CAD build for the part. Positions are in the model's coordinates, mm. A direction names the side the tool comes from. Coordinates: 2 decimals unless noted, no trailing zeros. Loops run counter-clockwise (first coordinate to the right, second up) from the corner with the lowest first, then second, coordinate; pieces in that order, holes last. Notation, with made-up numbers: M 12,82 L 39,82 A5 cw 39,91 Z; hole C 82.25,-30.5 d7. An arc over 180 degrees is marked long. Answer as a JSON object with one key per item and string values. Group by question number.
Solid Edge part; units mm, degrees
sketch "Sketch1" plane through (0, 0, 0) normal (0, -1, 0) x (1, 0, 0)
  line L0 (139.7, 114.3) -> (-139.7, 114.3)
  line L1 (-139.7, 114.3) -> (-139.7, -114.3)
  line L2 (-139.7, -114.3) -> (139.7, -114.3)
  line L3 (139.7, -114.3) -> (139.7, 114.3)
extrude "Protrusion1" add sketch "Sketch1" against normal blind 158.75
shell "Thinwall_1" thickness 38.1 removed faces 1 at (-90.3393, 0, 78.486)
Item 1: Slice it at B-B, the plane z = -41. Write the cut outline in (x, y).
Item 2: Pull direction Z, two halves, no side cores. Call faces 1 (the flat face through (2, 158.75, 2)), 2 (the flat face through (2, 78, 114.3)), 3 (the flat face through (101.6, 59, -1)): released by +Z, released by -Z, zero draft, split by the parting line, or undercut.
Item 3: Tool access for faces 4 (the flat face through (-1, 59, -76.2)), 5 (the flat face through (-2, 78, -114.3)): list every direction of +Z, -Z, +X, -X, +Y, -Y with a clear straight run to the whole face (end or side of a thin tool).
Item 4: Drill centre lines: L1, parallel to Z at x = 21, y = 90; L2, parallel to X at y = 7.5, z = 16.5; L3, parallel to Y at x = -3.5, z = -15. Where is each one in solid material? Low to high. Write a range as from..to.
Item 5: Slice it at C-C, the plane x = 45.5. Write the cut outline in (y, z).
Item 6: Slice it at A-A, the plane y = 84.5. Write the cut outline in (x, z).
Computed:
{
 "1": {"outline": "M -139.7,0 L -101.6,0 L -101.6,120.65 L 101.6,120.65 L 101.6,0 L 139.7,0 L 139.7,158.75 L -139.7,158.75 Z"},
 "2": {"face 1": "zero draft", "face 2": "released by +Z", "face 3": "undercut"},
 "3": {"face 4": "-Y", "face 5": "-Z, +X, -X, +Y, -Y"},
 "4": {"L1": "-114.3..-76.2, 76.2..114.3", "L2": "-139.7..-101.6, 101.6..139.7", "L3": "120.65..158.75"},
 "5": {"outline": "M 0,-114.3 L 158.75,-114.3 L 158.75,114.3 L 0,114.3 L 0,76.2 L 120.65,76.2 L 120.65,-76.2 L 0,-76.2 Z"},
 "6": {"outline": "M -139.7,-114.3 L 139.7,-114.3 L 139.7,114.3 L -139.7,114.3 Z; hole M -101.6,-76.2 L 101.6,-76.2 L 101.6,76.2 L -101.6,76.2 Z"}
}
